Print and shaded views of the part. All mm, measured from the part's lowest x, y and z. A direction names the side the tool comes from. Give positions to 0.01 mm unless a question says otherwise; leave off trailing zeros. Write each loop counter-clockwise with the first axis right and the second up, starting at its lowest first coordinate (ties: lowest second). Pieces come first, ordered by that corner, then holes. Notation, with made-up numbers: (42, 58.25) -> (59, 58.25) arc R20 cw to (59, 66.25) -> close; hole circle Ø11 at (59, 56.25). An arc over 180 degrees is marked (long way). Put each result on its own line as item: value.
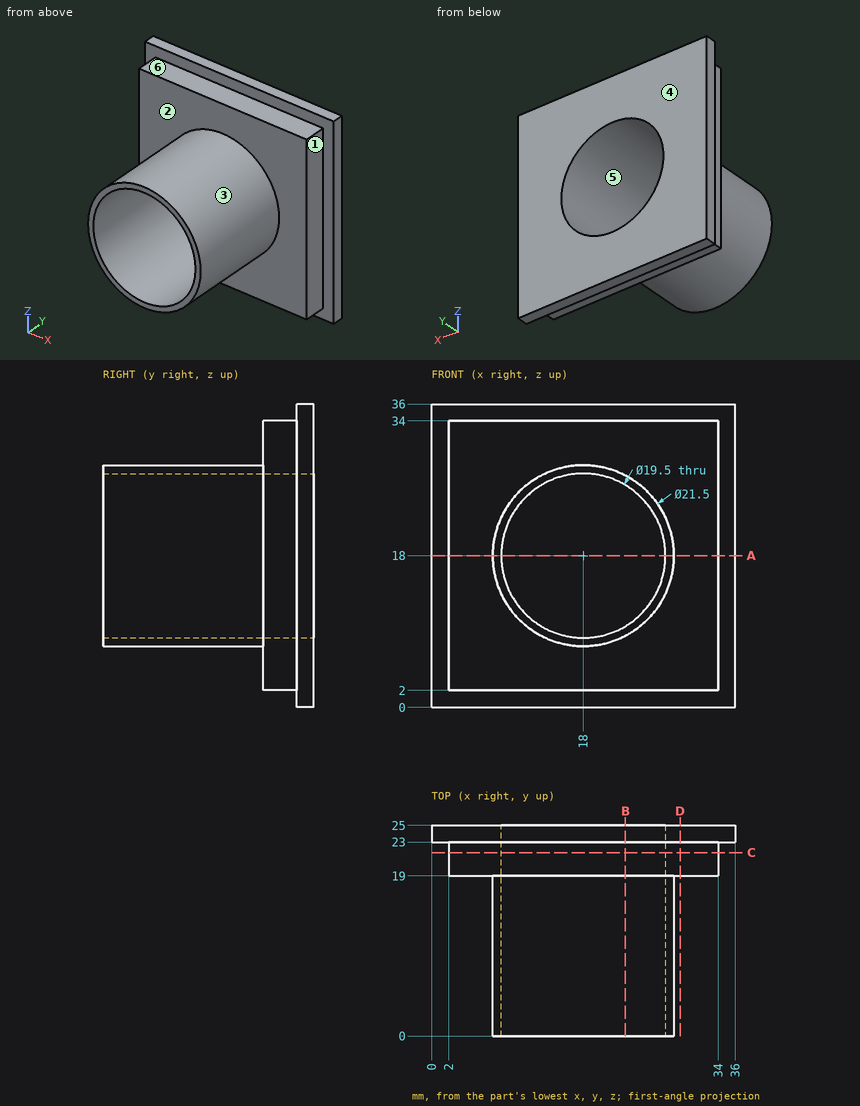
1) Slice it at B-B (x = 23). Write the cut outline in (y, z).
Filled sheet:
outline: (0, 8.48) -> (19, 8.48) -> (19, 2) -> (23, 2) -> (23, 0) -> (25, 0) -> (25, 9.63) -> (0, 9.63) -> close; (0, 26.37) -> (25, 26.37) -> (25, 36) -> (23, 36) -> (23, 34) -> (19, 34) -> (19, 27.52) -> (0, 27.52) -> close
2) Pull direction Z, two halves, no side cores. Call the marked faces 3, 4, 5 and 6: released by +Z, released by -Z, zero draft, split by the parting line, or undercut.
Filled sheet:
face 3: split by the parting line
face 4: zero draft
face 5: undercut
face 6: released by +Z
3) Slice it at A-A (z = 18). Write the cut outline in (x, y).
Filled sheet:
outline: (0, 23) -> (2, 23) -> (2, 19) -> (7.25, 19) -> (7.25, 0) -> (8.25, 0) -> (8.25, 25) -> (0, 25) -> close; (27.75, 0) -> (28.75, 0) -> (28.75, 19) -> (34, 19) -> (34, 23) -> (36, 23) -> (36, 25) -> (27.75, 25) -> close
4) Slice it at D-D (x = 29.5). Write the cut outline in (y, z).
Filled sheet:
outline: (19, 2) -> (23, 2) -> (23, 0) -> (25, 0) -> (25, 36) -> (23, 36) -> (23, 34) -> (19, 34) -> close
5) Wall check: L1, parallel to Z at x = 18, y = 6.5; L2, parallel to Y at x = 31.5, z = 18; L3, parallel to X at y = 18, z = 22. Give the ranges that are in metal, low to high.
Filled sheet:
L1: 7.25 to 8.25, 27.75 to 28.75
L2: 19 to 25
L3: 8.02 to 9.11, 26.89 to 27.98
6) Tool access for the marked faces 1 and 2: list every direction of +Z, -Z, +X, -X, +Y, -Y with a clear straight run to the whole face (end or side of a thin tool).
Filled sheet:
face 1: +Z, -Z, +X, -Y
face 2: -Y
7) Slice it at C-C (y = 21.75). Write the cut outline in (x, z), plus the area to 3 significant figures.
Filled sheet:
outline: (2, 2) -> (34, 2) -> (34, 34) -> (2, 34) -> close; hole circle Ø19.5 at (18, 18)
area: 725 mm2
8) Pin check, flat tips, straight feed: pin 1 (1 mm diameter, centred on x = 15.5, z = 5.5, fed in from -Y); pin 2 (2 mm diameter, centred on y = 21, z = 25, fed in from -X); pin 3 (1.5 mm diameter, centred on x = 13, y = 16.5, fed in from -Z); pin 4 (3 mm diameter, centred on x = 17.5, z = 25.5, fed in from -Y). Stop position of each tip, or through.
Filled sheet:
pin 1: y = 19
pin 2: x = 2
pin 3: z = 8.13
pin 4: through
